Check sheet for the drawn part. Datum: minimum x, y, z corner. Units: mm. A direction names the side the tool comes from. Give positions to 0.01 mm unless a question says otherwise; leave off trailing zeros. Order: outer loops, then holes, each group sorted by start corner. A loop starts at its lowest first (then second) coordinate and runs counter-clockwise, first axis right, second up.
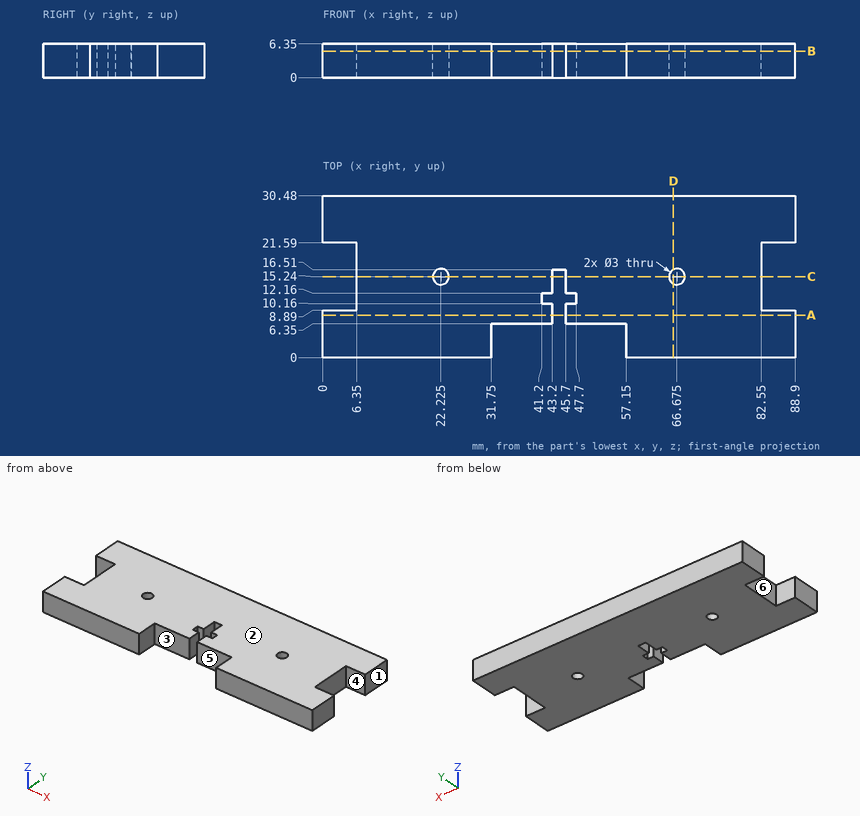
Item 1: Draft check along X on the marked faces 1, 2 and 3. Enter one of: released by +X, released by -X, zero draft, split by the parting line, or undercut.
Reported:
face 1: released by +X
face 2: zero draft
face 3: undercut
Item 2: Sectioned sample at D-D (x = 66). Enter the section's corners in (y, z).
Reported:
outline: (0, 0) - (13.9, 0) - (13.9, 6.35) - (0, 6.35) - close; (16.58, 0) - (30.48, 0) - (30.48, 6.35) - (16.58, 6.35) - close
Item 3: Set-up check for the marked faces 4, 5 and 6: record each of +Z, -Z, +X, -X, +Y, -Y from which the full face is reachable in a straight line by a thin tool's end or side.
Reported:
face 4: +Z, -Z, +X
face 5: +Z, -Z, -Y
face 6: +Z, -Z, -X
Item 4: Sectioned sample at A-A (y = 8). Enter the section's corners in (x, z), and give its area (3 significant figures).
Reported:
outline: (0, 0) - (43.2, 0) - (43.2, 6.35) - (0, 6.35) - close; (45.7, 0) - (88.9, 0) - (88.9, 6.35) - (45.7, 6.35) - close
area: 549 mm2
Item 5: Sectioned sample at B-B (z = 5). Give the number of separate pieces and of enclosed holes in the cut face, and give its area (3 significant figures).
Reported:
separate pieces: 1
enclosed holes: 2
area: 2,340 mm2
Item 6: Sectioned sample at C-C (y = 15.24). Enter the section's corners in (x, z) (3 decimals), and give its area (3 significant figures).
Reported:
outline: (6.35, 0) - (20.725, 0) - (20.725, 6.35) - (6.35, 6.35) - close; (23.725, 0) - (43.2, 0) - (43.2, 6.35) - (23.725, 6.35) - close; (45.7, 0) - (65.175, 0) - (65.175, 6.35) - (45.7, 6.35) - close; (68.175, 0) - (82.55, 0) - (82.55, 6.35) - (68.175, 6.35) - close
area: 430 mm2
Item 7: Gauge pin test, flat ends, axial feed: pin 1 (2 mm diameter, centred on y = 11, z = 4.5, fed in from -X); pin 2 (4 mm diameter, centred on x = 66.675, y = 15.24, fed in from -Z); pin 3 (1.6 mm diameter, centred on x = 47, z = 3.5, fed in from -Y); pin 4 (1 mm diameter, centred on y = 10.5, z = 3, fed in from +X). Record the tip position at first contact, or that the pin passes through.
Reported:
pin 1: stops at x = 6.35
pin 2: stops at z = 0
pin 3: stops at y = 6.35
pin 4: stops at x = 82.55
Item 8: Scan lines: L1, parallel to X at y = 5, z = 3.75; L2, parallel to X at y = 7, z = 3.5; L3, parallel to X at y = 20, z = 1. Record each from-to range of solid material in increasing order.
Reported:
L1: x = 0 to 31.75, 57.15 to 88.9
L2: x = 0 to 43.2, 45.7 to 88.9
L3: x = 6.35 to 82.55
